Input: part model. Units: mm. Frame: model coordinates. A direction names the side the tool comes from. Coordinates: 2 decimals unless noted, no trailing zeros. Write each loop counter-clockwise with the first axis right and the second up, starting at its lowest first coordinate (ties: lowest second). Pieces come first, ordered by that corner, then holes.
1) Line query: L1, parallel to X at y = -7.5, z = 4.9; L2, parallel to Y at x = 0, z = 2.7; L3, parallel to Z at x = -6, y = -12.5. Output: solid intervals per line, ascending.
2) Section query B-B (z = 6.25). Output: boundary loops of the cut face in (x, y), then the cut area to 3 significant figures.
3) Section query C-C (y = -14). Output: boundary loops of the cut face in (x, z).
4) Pin query (flat end, axial travel): pin 1 Ø2.5 at (y, z) = (-10, 5.5) entering from +X; pin 2 Ø1.4 at (x, y) = (7.5, -8) entering from +Z. Return the tip coordinate at first contact, or that it passes through.
5) Set-up query: faces 1 (the flat face through (0, -11.45, -1)), 2 (the flat face through (-7, -7, 2.5)), 3 (the flat face through (9.7, -7, 2)), 4 (the flat face through (4.88, -7, 5)). Return all of +Z, -Z, +X, -X, +Y, -Y with unobstructed straight access to the full face (end or side cutting, diameter ignored); none if empty.
6) Section query A-A (x = 0). Output: boundary loops of the cut face in (y, z), then the cut area to 3 significant figures.
7) Section query D-D (y = -7.25). Output: boundary loops of the cut face in (x, z).
8) Draft query along Y for faces 5 (the flat face through (3.437, -9.447, -0.528)), 6 (the flat face through (-3, -4, -2.5)), 7 (the flat face through (0, 0, 3)). Return one class per face: pulls with the +Y half, pulls with the -Y half, needs draft (parallel to the pull), parting line crosses it, or undercut.
from build123d import *

# Parameters (mm, degrees)
F0_W     = 9.76
F0_H     = 5
F1_DEPTH = 15
F2_SIZE  = 3.2
F3_R     = 2.65
F4_DEPTH = 10.001
F5_DEPTH = 4
F6_R     = 1


with BuildPart() as f1:
    # F0 (on Front) → F1 (new body)
    with BuildSketch(Plane.XZ):
        Polygon((-9.7, -2.5), (9.7, -2.5), (9.7, 2.5), (4.88, 2.5), (-4.88, 2.5), (-9.7, 2.5), align=None)
        with Locations((0, 5)):
            Rectangle(F0_W, F0_H)
    extrude(amount=F1_DEPTH)

    # F2
    f2_edges = [f1.edges().sort_by_distance(p)[0] for p in [
        (9.7, -7.5, -2.5),
        (-9.7, -7.5, -2.5),
    ]]
    chamfer(f2_edges, length=F2_SIZE)

    # F3 (on face) → F4 (cut, through all)
    with BuildSketch(Plane(origin=(0, 0, -2.5), x_dir=(1, 0, 0), z_dir=(0, 0, -1))):
        with Locations((0, 7.5)):
            Circle(F3_R)
    extrude(amount=-F4_DEPTH, mode=Mode.SUBTRACT)

    # F3 (on face) → F5 (cut)
    with BuildSketch(Plane(origin=(0, 0, -2.5), x_dir=(1, 0, 0), z_dir=(0, 0, -1))):
        Polygon((-2.2805335633, 3.55), (2.2805335633, 3.55), (4.5610671266, 7.5), (2.2805335633, 11.45), (-2.2805335633, 11.45), (-4.5610671266, 7.5), align=None)
        with Locations((0, 7.5)):
            Circle(F3_R, mode=Mode.SUBTRACT)
    extrude(amount=-F5_DEPTH, mode=Mode.SUBTRACT)

    # F6
    f6_edges = [f1.edges().sort_by_distance(p)[0] for p in [
        (-6.5, -7.5, -2.5),
        (6.5, -7.5, -2.5),
        (9.7, -7.5, 0.7),
        (-9.7, -7.5, 0.7),
    ]]
    fillet(f6_edges, radius=F6_R)


solid = f1.part
Answer:
1. L1: x = -4.88 to -2.65, 2.65 to 4.88
1. L2: y = -15 to -10.15, -4.85 to 0
1. L3: z = -2.5 to 2.5
2. outline: (-4.88, -15) - (4.88, -15) - (4.88, 0) - (-4.88, 0) - close; hole circle Ø5.3 at (0, -7.5)
2. area: 124 mm2
3. outline: (-9.7, 1.11) arc R1 ccw to (-9.41, 0.41) - (-6.79, -2.21) arc R1 ccw to (-6.09, -2.5) - (6.09, -2.5) arc R1 ccw to (6.79, -2.21) - (9.41, 0.41) arc R1 ccw to (9.7, 1.11) - (9.7, 2.5) - (4.88, 2.5) - (4.88, 7.5) - (-4.88, 7.5) - (-4.88, 2.5) - (-9.7, 2.5) - close
4. pin 1: stops at x = 4.88
4. pin 2: stops at z = 2.5
5. face 1: -Z
5. face 2: +Z, -X, +Y, -Y
5. face 3: +Z, -Z, +X, +Y, -Y
5. face 4: +Z, +X, +Y, -Y
6. outline: (-15, -2.5) - (-11.45, -2.5) - (-11.45, 1.5) - (-10.15, 1.5) - (-10.15, 7.5) - (-15, 7.5) - close; (-4.85, 1.5) - (-3.55, 1.5) - (-3.55, -2.5) - (0, -2.5) - (0, 7.5) - (-4.85, 7.5) - close
6. area: 86.6 mm2
7. outline: (-9.7, 1.11) arc R1 ccw to (-9.41, 0.41) - (-6.79, -2.21) arc R1 ccw to (-6.09, -2.5) - (-4.42, -2.5) - (-4.42, 1.5) - (-2.64, 1.5) - (-2.64, 7.5) - (-4.88, 7.5) - (-4.88, 2.5) - (-9.7, 2.5) - close; (2.64, 1.5) - (4.42, 1.5) - (4.42, -2.5) - (6.09, -2.5) arc R1 ccw to (6.79, -2.21) - (9.41, 0.41) arc R1 ccw to (9.7, 1.11) - (9.7, 2.5) - (4.88, 2.5) - (4.88, 7.5) - (2.64, 7.5) - close
8. face 5: undercut
8. face 6: needs draft
8. face 7: pulls with the +Y half
